```python
from build123d import *

# Parameters (mm, degrees)
BOSS_EXTRUDE1_DEPTH = 7
BOSS_EXTRUDE2_DEPTH = 7
FILLET1_R           = 7
CUT_EXTRUDE1_REACH  = 66.771
SKETCH6_R           = 4


with BuildPart() as part:
    # Sketch1 → Boss-Extrude1 (new body)
    with BuildSketch(Plane.XY):
        Polygon((-44, 25), (-38, 31), (38, 31), (44, 25), (44, -25), (38, -31), (-38, -31), (-44, -25), align=None)
        with BuildLine():
            Line((-31.385621722, 20.5), (-31.385621722, -20.5))
            ThreePointArc((-31.385621722, -20.5), (-34.385621722, -23.5), (-37.385621722, -20.5))
            Line((-37.385621722, -20.5), (-37.385621722, 20.5))
            ThreePointArc((-37.385621722, 20.5), (-34.385621722, 23.5), (-31.385621722, 20.5))
        make_face(mode=Mode.SUBTRACT)
        with BuildLine():
            Line((31.385621722, 20.5), (31.385621722, -20.5))
            ThreePointArc((31.385621722, -20.5), (34.385621722, -23.5), (37.385621722, -20.5))
            Line((37.385621722, -20.5), (37.385621722, 20.5))
            ThreePointArc((37.385621722, 20.5), (34.385621722, 23.5), (31.385621722, 20.5))
        make_face(mode=Mode.SUBTRACT)
    extrude(amount=BOSS_EXTRUDE1_DEPTH)

    # Sketch2 → Boss-Extrude2 (add, symmetric)
    with BuildSketch(Plane(origin=(0, 0, 0), x_dir=(-0.8589373126285005, 0.5120807484904403, 0), z_dir=(-0.5120807484904403, -0.8589373126285005, 0))):
        Polygon((20.032748859, 0), (-14.300096017, 0), (-14.300096017, 20), (-26.435350933, 28.816778784), (-24.084209923, 32.052846762), (-14.300096017, 24.94427191), align=None)
    extrude(amount=BOSS_EXTRUDE2_DEPTH, both=True)

    # Fillet1
    fillet1_edges = [part.edges().sort_by_distance(p)[0] for p in [
        (25.281133158, -6.92248608, -30.434812773),
        (18.112002679, -18.947608457, -30.434812773),
    ]]
    fillet(fillet1_edges, radius=FILLET1_R - 0.0001)  # a hair under: the kernel refuses the full size

    # Sketch6 → Cut-Extrude1 (cut, up to next)
    with BuildSketch(Plane(origin=(-5.944829265, 3.544184861, -9.526138171), x_dir=(-0.8631949903821312, -0.17604689815365596, 0.4731827323874666), z_dir=(-0.5048706850067575, 0.30099351194556917, -0.8090169943749512)), mode=Mode.PRIVATE) as cut_extrude1_sk1:
        with Locations(Location((-25.217235821, -18.583042284, 0), (0, 0, 10.638271161))):
            Circle(SKETCH6_R)
    cut_extrude1_tool1 = extrude(cut_extrude1_sk1.sketch, amount=-CUT_EXTRUDE1_REACH, mode=Mode.PRIVATE) & part.part
    add(cut_extrude1_tool1.solids().sort_by_distance((15.822562, -9.433086, -27.93835))[0], mode=Mode.SUBTRACT)


solid = part.part
```
Here's how the part is built. I have some questions about the finished solid (model axes, mm). A direction names the side the tool comes from. Give positions to 0.01 mm unless a question says otherwise; leave off trailing zeros. Write each loop counter-clockwise with the first axis right and the second up, starting at its lowest first coordinate (ties: lowest second). Pieces come first, ordered by that corner, then holes. Notation, with made-up numbers: (33, 24) -> (81, 24) arc R13 cw to (81, 42) -> close; hole circle Ø4 at (86, 37). An arc over 180 degrees is marked (long way). Use one line per item in the form item = value.
1) I'm going to push flat-ended pins straight in: pin 1 (5 mm diameter, centred on x = -7.5, z = -10, fed in from -Y); pin 2 (3 mm diameter, centred on y = 5.5, z = -8, fed in from -X); pin 3 (12 mm diameter, centred on x = 3, z = -15, fed in from +Y). Where does each tip first touch, or does it pass through?
Verdict:
pin_1 = -5.17
pin_2 = -9.79
pin_3 = 8.8
2) Suppose I cut it at C-C (y = -8). Give the number of separate pieces and of enclosed holes in the cut face, and give its area (3 significant figures).
Verdict:
separate_pieces = 4
enclosed_holes = 0
area = 815 mm2
3) Suppose I cut it at D-D (z = -4.5). Please give me the cut outline in (x, y).
Verdict:
outline = (-15.47, 1.07) -> (8.7, -13.34) -> (15.87, -1.31) -> (-8.3, 13.1) -> close
4) Suppose I cut it at A-A (x = 35). Please give me the cut outline in (y, z).
Verdict:
outline = (-31, 0) -> (-23.44, 0) -> (-23.44, 7) -> (-31, 7) -> close; (23.44, 0) -> (31, 0) -> (31, 7) -> (23.44, 7) -> close
5) On a 3-axis mill with a long thin cutter (end or side, diameter ignored), from which of +Z, -Z, +X, -X, +Y, -Y can I reach the whole of each face in a straight line? I mean faces 1 (the face through (15.852, -7.754, -22.387)), 2 (the face through (-41, -28, 3)), 3 (the face through (-34.3, -23.5, 3.5)). Say none if no direction works.
Verdict:
face_1 = +X, -Y
face_2 = +Z, -Z, -X, -Y
face_3 = +Z, -Z
6) If I drill on L1, parallel to Z at x = 22.5, y = -4.5; L2, parallel to X at y = 21, z = 5.5; L3, parallel to Y at x = 32.5, z = 0.5, over which ranges is the centre line in solid material (lowest first)? Write a range as [from, to].
Verdict:
L1 = [0, 7]
L2 = [-44, -37.34], [-31.43, 31.43], [37.34, 44]
L3 = [-31, -22.83], [22.83, 31]
7) Suppose I cut it at B-B (x = -27.5). Please give me the cut outline in (y, z), and give its area (3 significant figures).
Verdict:
outline = (-31, 0) -> (31, 0) -> (31, 7) -> (-31, 7) -> close
area = 434 mm2
8) We'd pull the mould along Z, two halves only. Please class faces 4 (the face through (12.23, -7.41, -9.86)), 5 (the face through (20.24, -9.86, -28.41)), 6 (the face through (1, -31, 3)), 7 (the face through (1, 0, 7)): +Z half, -Z half, draft (parallel to the pull), parting line (faces both ways), or undercut.
Verdict:
face_4 = undercut
face_5 = undercut
face_6 = draft
face_7 = +Z half
